Input: part model. Units: mm. Frame: model coordinates. A direction names the side the tool comes from. Give positions to 0.01 mm unless a question says otherwise; leave off trailing zeros. Loops run counter-clockwise (first coordinate to the right, second up) from the corner with the lowest first, then second, coordinate; pieces in that order, holes last. Notation, with made-up numbers: M 2.5,-24.75 L 25.5,-24.75 A19 cw 25.5,-17.75 Z; hole C -15,56.5 d4. An arc over 180 degrees is marked long. One line per item, written item: value. Start each with the question number.
(1) Section B-B on x = 0. State how many separate pieces and enclosed holes the cut face has, plus the area to 3 significant figures.
(2) Section C-C on z = 15. Output: boundary loops of the cut face in (x, y), plus the area to 3 significant figures.
(3) Access query for faces 1 (the flat face through (-5, -6, 5)), 2 (the cylindrical face through (-26, 0, 5)). Directions: +Z, -Z, +X, -X, +Y, -Y. A direction counts if a zero-diameter tool reaches every point of the face in a straight line with its end or side. Return the directions, or none.
(4) Ray query, line 1 along Z through (x, y) = (0, -9.7); line 2 along Y through (x, z) = (-15, 3.75); line 3 along Y through (x, z) = (-14, 12.5). Return the intervals inside material, ascending. Write a range as from..to.
(5) Pin query (flat end, axial travel): P1, Ø5, axis at x = 0, z = 15, coming from the +Y side; P2, Ø4, axis at x = -6.5, y = -2.5, coming from the +Z side; P3, Ø3, axis at x = 20.5, y = 5.5, coming from the +Z side; P4, Ø4, axis at y = 3, z = 3, coming from the -X side. Return the tip coordinate at first contact, or that it passes through.
(6) Pull-direction query (Z, two-part tool) for faces 3 (the cylindrical face through (-0.521, -9.521, 18.966)), 4 (the flat face through (0, -11, 9)), 5 (the cylindrical face through (-0.1, -9.5, 22.5)); classes: released by +Z, released by -Z, zero draft, split by the parting line, or undercut.
(7) Section D-D on y = 0. Output: boundary loops of the cut face in (x, z).
(8) Section A-A on z = 1.75. Output: boundary loops of the cut face in (x, y), plus the area to 3 significant figures.
```python
from build123d import *

# Parameters (mm, degrees)
F0_R     = 3.0896655398
F1_DEPTH = 25
F2_R     = 4
F3_DEPTH = 25
F6_DEPTH = 25
F7_R     = 0.99999


# Not quite as in the source:
# - a fillet or chamfer is up to 0.001 mm smaller than in the source, because OpenCascade refuses the exact size


with BuildPart() as f1:
    # F0 (on Top) → F1 (new body)
    with BuildSketch(Plane.XY):
        with BuildLine():
            ThreePointArc((-15, 11), (-26, 0), (-15, -11))
            Line((-15, -11), (15, -11))
            ThreePointArc((15, -11), (26, 0), (15, 11))
            Line((15, 11), (-15, 11))
        make_face()
        with Locations((-15, 0)):
            Circle(F0_R, mode=Mode.SUBTRACT)
        with BuildLine():
            ThreePointArc((7, 0), (0, -7), (-7, 0))
            ThreePointArc((-7, 0), (0, 7), (7, 0))
        make_face(mode=Mode.SUBTRACT)
        with BuildLine():
            ThreePointArc((18.1, 0), (15, -3.1), (11.9, 0))
            ThreePointArc((11.9, 0), (15, 3.1), (18.1, 0))
        make_face(mode=Mode.SUBTRACT)
    extrude(amount=F1_DEPTH)

    # F2 (on face) → F3 (cut)
    with BuildSketch(Plane.XZ.offset(11)):
        with BuildLine():
            Line((15, 25), (-15, 25))
            Line((-15, 25), (-15, 13.6771502157))
            Line((-15, 13.6771502157), (-4.2923891696, 21.1502353789))
            ThreePointArc((-4.2923891696, 21.1502353789), (0, 22.5), (4.2923891696, 21.1502353789))
            Line((4.2923891696, 21.1502353789), (15, 13.6771502157))
            Line((15, 13.6771502157), (15, 25))
        make_face()
        with BuildLine():
            Line((26, 25), (-26, 25))
            Line((-26, 25), (-26, 6))
            Line((-26, 6), (-4.2923891696, 21.1502353789))
            ThreePointArc((-4.2923891696, 21.1502353789), (0, 22.5), (4.2923891696, 21.1502353789))
            Line((4.2923891696, 21.1502353789), (26, 6))
            Line((26, 6), (26, 25))
        make_face()
        with Locations((0, 15)):
            Circle(F2_R)
    extrude(amount=-F3_DEPTH, mode=Mode.SUBTRACT)

    # F5 (on offset) → F6 (cut)
    with BuildSketch(Plane(origin=(0, 0, 5), x_dir=(1, 0, 0), z_dir=(0, 0, -1))):
        with BuildLine():
            Line((-15, -8), (15, -8))
            ThreePointArc((15, -8), (23, 0), (15, 8))
            Line((15, 8), (-15, 8))
            ThreePointArc((-15, 8), (-23, 0), (-15, -8))
        make_face()
    extrude(amount=-F6_DEPTH, mode=Mode.SUBTRACT)

    # F7 (radius 1 in the source; OpenCascade refuses exactly that, so slightly less here)
    f7_edges = [f1.edges().sort_by_distance(p)[0] for p in [
        (0, -8, 5),
    ]]
    fillet(f7_edges, radius=F7_R)


solid = f1.part
```
Output values:
1. separate pieces: 4
1. enclosed holes: 0
1. area: 97.4 mm²
2. outline: M -13.1,-11 L -4,-11 L -4,-8 L -13.1,-8 Z; M -13.1,8 L -4,8 L -4,11 L -13.1,11 Z; M 4,-11 L 13.1,-11 L 13.1,-8 L 4,-8 Z; M 4,8 L 13.1,8 L 13.1,11 L 4,11 Z
2. area: 109 mm²
3. face 1: +Z
3. face 2: +Z, -Z, -X
4. line 1: z = 0..11, 19..22.5
4. line 2: y = -11..-3.09, 3.09..11
4. line 3: y = -11..-8, 8..11
5. P1: passes through
5. P2: stops at z = 5
5. P3: stops at z = 10.54
5. P4: stops at x = -25.95
6. face 3: undercut
6. face 4: zero draft
6. face 5: released by +Z
7. outline: M -26,0 L -18.09,0 L -18.09,5 L -22,5 A1 cw -23,6 L -23,8.09 L -26,6 Z; M -11.91,0 L -7,0 L -7,5 L -11.91,5 Z; M 7,0 L 11.9,0 L 11.9,5 L 7,5 Z; M 18.1,0 L 26,0 L 26,6 L 23,8.09 L 23,6 A1 cw 22,5 L 18.1,5 Z
8. outline: M -15,-11 L 15,-11 A11 ccw 15,11 L -15,11 A11 ccw Z; hole C -15,0 d6.18; hole C 0,0 d14; hole C 15,0 d6.2
8. area: 826 mm²
